Autodesk Inventor part; units mm, degrees
ref_plane "YZ Plane" through (0, 0, 0) normal (1, 0, 0) x (0, 1, 0)
ref_plane "XZ Plane" through (0, 0, 0) normal (0, 1, 0) x (-1, 0, 0)
ref_plane "XY Plane" through (0, 0, 0) normal (0, 0, 1) x (1, 0, 0)
sketch "Skizze1" plane through (0, 0, 0) normal (0, 1, 0) x (-1, 0, 0)
  line L0 (49, 0) -> (-49, 0)
  line L1 (0, -66.5) -> (0, 66.5)
  line L2 (-35, 47.5) -> (35, 47.5)
  line L3 (35, 47.5) -> (35, -47.5)
  line L4 (35, -47.5) -> (-35, -47.5)
  line L5 (-35, -47.5) -> (-35, 47.5)
  point P0 (0, 0)
  dimension "d0" = 70
  dimension "d1" = 95
extrude "Extrusion1" add sketch "Skizze1" along normal blind 1
sketch "Skizze2" plane through (0, 1, 0) normal (0, 1, 0) x (1, 0, 0)
  line L0 (-35, -47.5) -> (35, -47.5)
  line L1 (35, -47.5) -> (35, 47.5)
  line L2 (35, 47.5) -> (-35, 47.5)
  line L3 (-35, 47.5) -> (-35, -47.5)
  line L4 (-33.9, 46.4) -> (33.9, 46.4)
  line L5 (33.9, 46.4) -> (33.9, -46.4)
  line L6 (33.9, -46.4) -> (-33.9, -46.4)
  line L7 (-33.9, -46.4) -> (-33.9, 46.4)
  point P0 (0, 0)
  dimension "d4" = 1.1
extrude "Extrusion2" add sketch "Skizze2" along normal blind 40
properties part number "Boden" material "ABS-Kunststoff"
Here's how the part is built. I have some questions about the finished solid (model axes, mm). A direction names the side the tool comes from. Round coordinates to 2 decimals unless told otherwise and drop trailing zeros. Write each loop counter-clockwise with the first axis right and the second up, starting at its lowest first coordinate (ties: lowest second). Pieces come first, ordered by that corner, then holes.
Q1. If we mould it in two halves opening along X, with no side actions, what happens to faces 3 (the flat face through (33.9, 21, -1)), 4 (the flat face through (0, 0, 1)), 5 (the flat face through (-35, 20, -1)), 6 (the flat face through (-33.9, 21, 1))? For each: +X half, -X half, draft (parallel to the pull), parting line (faces both ways), or undercut.
Q2. If we section it at B-B on y = 8: Write out the boundary of the cut face in (x, z), plus the area to 3 significant figures.
Q3. If we section it at A-A on z = 3: Write out the boundary of the cut face in (x, y), plus the area to 3 significant figures.
Q4. Which directions (+Z, -Z, +X, -X, +Y, -Y) give clear straight access to the entire face, cutting with the end or side of a thin tool? Please do faces 1 (the flat face through (0, 20, -47.5)), 2 (the flat face through (0, 21, -46.4)).
Q5. Please list where these lines run through material, in increasing order: probe 1 along Z at (x, y) = (-19.5, 9); probe 2 along X at (y, z) = (22, 33); probe 3 along Y at (x, z) = (2.5, -43).
Q6. Will this pin go through, and if not, where does the flat tip stop? P1, Ø2, axis at x = 11, z = -3, coming from the +Y side.
Q7. If we section it at C-C on x = -27: Write out the boundary of the cut face in (y, z), plus the area to 3 significant figures.
Answer below:
1. face 3: undercut
1. face 4: draft
1. face 5: -X half
1. face 6: undercut
2. outline: (-35, -47.5) - (35, -47.5) - (35, 47.5) - (-35, 47.5) - close; hole (-33.9, -46.4) - (33.9, -46.4) - (33.9, 46.4) - (-33.9, 46.4) - close
2. area: 358 mm2
3. outline: (-35, 0) - (35, 0) - (35, 41) - (33.9, 41) - (33.9, 1) - (-33.9, 1) - (-33.9, 41) - (-35, 41) - close
3. area: 158 mm2
4. face 1: -Z, +X, -X, +Y, -Y
4. face 2: +Y
5. probe 1: z = -47.5 to -46.4, 46.4 to 47.5
5. probe 2: x = -35 to -33.9, 33.9 to 35
5. probe 3: y = 0 to 1
6. P1: stops at y = 1
7. outline: (0, -47.5) - (41, -47.5) - (41, -46.4) - (1, -46.4) - (1, 46.4) - (41, 46.4) - (41, 47.5) - (0, 47.5) - close
7. area: 183 mm2
